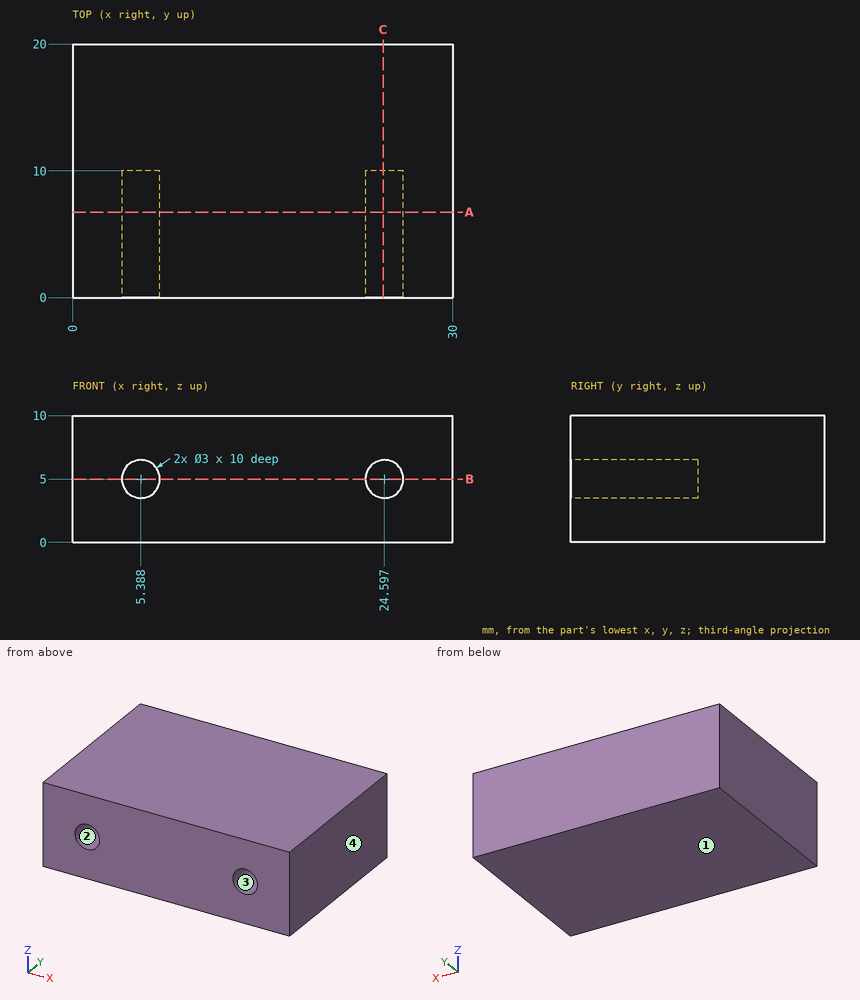
Design review of the part shown in the three views and the two pictorial views. Dimensions are in mm from the part's minimum x, y and z. Give positions to 0.01 mm unless a question says otherwise; leave off trailing zeros. Write each loop counter-clockwise with the first axis right and the second up, starting at its lowest first coordinate (ties: lowest second). Pieces come first, ordered by that corner, then holes.
(1) Add section A-A (y = 6.75). Give the boundary of the cut face in (x, z), and give its area (3 significant figures).
Checked values:
outline: (0, 0) - (30, 0) - (30, 10) - (0, 10) - close; hole circle Ø3 at (5.39, 5); hole circle Ø3 at (24.6, 5)
area: 286 mm2
(2) Wall thickness on line 1 along Z through (x, y) = (6.5, 9.5) (1 decimal): over which ranges is the line inside the solid? List them lowest first.
Checked values:
line 1: z = 0 to 4, 6 to 10
(3) Add section B-B (z = 5). Give the boundary of the cut face in (x, y), and give its area (3 significant figures).
Checked values:
outline: (0, 0) - (3.89, 0) - (3.89, 10) - (6.89, 10) - (6.89, 0) - (23.1, 0) - (23.1, 10) - (26.1, 10) - (26.1, 0) - (30, 0) - (30, 20) - (0, 20) - close
area: 540 mm2
(4) Add section C-C (x = 24.5). Give the boundary of the cut face in (y, z), and give its area (3 significant figures).
Checked values:
outline: (0, 0) - (20, 0) - (20, 10) - (0, 10) - (0, 6.5) - (10, 6.5) - (10, 3.5) - (0, 3.5) - close
area: 170 mm2
(5) Clearance check with a flat-ended pin moving along its axis: pin 1 Ø2.5 at (x, z) = (24.6, 5) entering from -Y. State where the tip first meets the part, or that it passes through.
Checked values:
pin 1: stops at y = 10
(6) Mouldability with a two-part tool opening along X and no side actions: class the marked faces 1, 2, 3 and 4 as +X half, -X half, draft (parallel to the pull), parting line (faces both ways), or undercut.
Checked values:
face 1: draft
face 2: undercut
face 3: undercut
face 4: +X half
